CAD build for the part. Positions are in the model's coordinates, mm. A direction names the side the tool comes from. Round coordinates to 2 decimals unless told otherwise and drop trailing zeros. Loops run counter-clockwise (first coordinate to the right, second up) from the corner with the lowest first, then second, coordinate; pieces in that order, holes last.
from build123d import *

# Parameters (mm, degrees)
SKETCH3_R          = 5
CUT_EXTRUDE1_DEPTH = 10


with BuildPart() as part:
    # Sketch2 → Revolve1 (revolve)
    with BuildSketch(Plane.XY, mode=Mode.PRIVATE) as revolve1_sk:
        Polygon((-47.527918782, 29.515656182), (-37.527918782, 29.515656182), (-37.527918782, 49.515656182), (-47.527918782, 49.515656182), (-47.527918782, 53.515656182), (-33.527918782, 53.515656182), (-33.527918782, 61.515656182), (-31.527918782, 61.515656182), (-29.384325242, 53.515656182), (-8.527918782, 53.515656182), (-8.527918782, 47.515656182), (-33.527918782, 47.515656182), (-33.527918782, 27.427572824), (-33.527918782, 25.515656182), (-47.527918782, 25.515656182), align=None)
    revolve(revolve1_sk.sketch.rotate(Axis((-68.527918782, 64.847715736, 0), (0, -1, 0)), 90), axis=Axis((-68.527918782, 64.847715736, 0), (0, -1, 0)))

    # Sketch3 → Cut-Extrude1 (cut)
    with BuildSketch(Plane(origin=(0, 53.515656182, 0), x_dir=(1, 0, 0), z_dir=(0, 1, 0))):
        with Locations(Location((-118.527918782, 0, 0), (0, 0, 270))):
            Circle(SKETCH3_R)
        with Locations(Location((-103.883257841, 35.355339059, 0), (0, 0, 270))):
            Circle(SKETCH3_R)
        with Locations(Location((-68.527918782, 50, 0), (0, 0, 270))):
            Circle(SKETCH3_R)
        with Locations(Location((-33.172579722, 35.355339059, 0), (0, 0, 270))):
            Circle(SKETCH3_R)
        with Locations(Location((-18.527918782, 0, 0), (0, 0, 270))):
            Circle(SKETCH3_R)
        with Locations(Location((-33.172579722, -35.355339059, 0), (0, 0, 270))):
            Circle(SKETCH3_R)
        with Locations(Location((-68.527918782, -50, 0), (0, 0, 270))):
            Circle(SKETCH3_R)
        with Locations(Location((-103.883257841, -35.355339059, 0), (0, 0, 270))):
            Circle(SKETCH3_R)
    extrude(amount=-CUT_EXTRUDE1_DEPTH, mode=Mode.SUBTRACT)


solid = part.part
Item 1: Cut at A-A (z = 50). List the corners of the cut face in (x, y).
Verdict:
outline: (-101.69, 47.52) - (-73.53, 47.52) - (-73.53, 53.52) - (-101.69, 53.52) - close; (-63.53, 47.52) - (-35.36, 47.52) - (-35.36, 53.52) - (-63.53, 53.52) - close
Item 2: Flat gauge pins, fed straight in: P1, Ø12, axis at y = 58, z = -2, coming from the -X side; P2, Ø5, axis at x = -74, y = 40.5, coming from the +Z side; P3, Ø2, axis at x = -67.5, y = 47, coming from the -Z side. Where does each tip first touch, or does it go through?
Verdict:
P1: stops at x = -128.53
P2: stops at z = 34.87
P3: stops at z = -60
Item 3: Cut at B-B (x = -21). List the corners of the cut face in (y, z), plus the area to 3 significant figures.
Verdict:
outline: (47.52, -36.62) - (53.52, -36.62) - (53.52, -4.35) - (47.52, -4.35) - close; (47.52, 4.35) - (53.52, 4.35) - (53.52, 36.62) - (47.52, 36.62) - close
area: 387 mm2
Item 4: 3-axis set-ups, long thin cutter, end or side, ignore diameter. For faces 1 (the flat face through (-53, 25.516, 15)), 2 (the cylindrical face through (-34.36, 36.67, -7.59)), 3 (the flat face through (-48, 29.516, -6)), 4 (the cylindrical face through (-73.41, 50.56, 48.92)), 5 (the cylindrical face through (-34.36, 57.57, -7.59)): which of +Z, -Z, +X, -X, +Y, -Y reach the whole face in a straight line?
Verdict:
face 1: +Z, -Z, +X, -X, -Y
face 2: -Y
face 3: none
face 4: +Y, -Y
face 5: +Y
Item 5: Cut at C-C (z = 0). State how many separate pieces and enclosed holes the cut face has, plus the area to 3 significant figures.
Verdict:
separate pieces: 4
enclosed holes: 0
area: 613 mm2
Item 6: Wall check: L1, parallel to X at y = 51, z = 0; L2, parallel to X at y = 27.35, z = 0; L3, parallel to Z at x = -37.5, y = 48. Give the ranges that are in metal, low to high.
Verdict:
L1: x = -128.53 to -123.53, -113.53 to -89.53, -47.53 to -23.53, -13.53 to -8.53
L2: x = -103.53 to -89.53, -47.53 to -33.53
L3: z = -51.35 to -37.86, -32.85 to 32.85, 37.86 to 51.35
Item 7: Mould opens along Z. For faces 6 (the cylindrical face through (-22.964, 50.558, 2.307)), 7 (the flat face through (-43, 47.516, 26)), 8 (the cylindrical face through (-89.35, 51.54, -2.73)), 9 (the conical face through (-35.584, 61.015, 17.135)) say: released by +Z, released by -Z, zero draft, split by the parting line, or undercut.
Verdict:
face 6: undercut
face 7: zero draft
face 8: undercut
face 9: split by the parting line
